Build history of the part. All positions in model axes, mm. Give positions to 0.01 mm unless a question says otherwise; leave off trailing zeros. Loops run counter-clockwise (first coordinate to the right, second up) from the corner with the lowest first, then second, coordinate; pieces in that order, holes last.
1) Wall check: line 1 (Z direction, x = 1.25, y = -9); line 2 (Y direction, x = 0.9, z = 7.75). Give the ranges that are in metal, low to high.
2) Flat gauge pins, fed straight in: P1, Ø3.5, axis at y = -9, z = -9, coming from the -X side; P2, Ø1.8, axis at y = 9, z = 9, coming from the +X side (3 decimals). Where does each tip first touch, or does it go through?
3) Band-saw the part on A-A on y = 9. List the corners of the cut face in (x, z).
4) Band-saw the part on C-C on x = 0.35. List the corners of the cut face in (y, z).
5) Two-plate mould, pull along Z, no slides. Class faces 1 (the flat face through (1.7, 0, 0)), 2 (the cylindrical face through (0.8, 7.8, 9.9)), 3 (the flat face through (1, 0, -11.5)): +Z half, -Z half, draft (parallel to the pull), parting line (faces both ways), or undercut.
Autodesk Inventor part; units mm, degrees
ref_plane "YZ Plane" through (0, 0, 0) normal (1, 0, 0) x (0, 1, 0)
ref_plane "XZ Plane" through (0, 0, 0) normal (0, 1, 0) x (-1, 0, 0)
ref_plane "XY Plane" through (0, 0, 0) normal (0, 0, 1) x (1, 0, 0)
sketch "Sketch1" plane through (0, 0, 0) normal (1, 0, 0) x (0, 1, 0)
  line L0 (11.5, 11.5) -> (-11.5, 11.5)
  line L1 (-11.5, 11.5) -> (-11.5, -11.5)
  line L2 (-11.5, -11.5) -> (11.5, -11.5)
  line L3 (11.5, -11.5) -> (11.5, 11.5)
  line L4 (11.5, 11.5) -> (-11.5, -11.5) construction
  line L5 (-11.5, 11.5) -> (11.5, -11.5) construction
  line L6 (11.5, 11.5) -> (11.5, 9)
  line L7 (11.5, 9) -> (9, 9)
  circle A0 centre (9, 9) radius 1.5
  line L8 (11.5, 0) -> (-11.5, 0)
  line L9 (0, 11.5) -> (0, -11.5)
  line L10 (11.5, -11.5) -> (-11.5, 11.5) construction
  line L11 (11.5, -9) -> (9, -9)
  circle A1 centre (9, -9) radius 1.5
  circle A2 centre (-9, 9) radius 1.5
  circle A3 centre (-9, -9) radius 1.5
  point P0 (0, 0)
  dimension "d0" = 23
  dimension "d1" = 23
  dimension "d2" = 2.5
  dimension "d3" = 2.5
  dimension "d4" = 3
extrude "Extrusion1" add sketch "Sketch1" along normal blind 1.7
ref_plane "Work Plane1" through (0, 0, 11.5) normal (0, 1, 0) x (1, 0, 0)
ref_plane "Work Plane2" through (0, -11.5, 0) normal (0, 0, -1) x (-1, 0, 0)
properties part number "magentic_encoder_modell"
Findings below:
1. line 1: z = -11.5 to -10.5, -7.5 to 7.5, 10.5 to 11.5
1. line 2: y = -11.5 to -9.83, -8.17 to 8.17, 9.83 to 11.5
2. P1: stops at x = 0
2. P2: passes through
3. outline: (0, -11.5) - (1.7, -11.5) - (1.7, -10.5) - (0, -10.5) - close; (0, -7.5) - (1.7, -7.5) - (1.7, 7.5) - (0, 7.5) - close; (0, 10.5) - (1.7, 10.5) - (1.7, 11.5) - (0, 11.5) - close
4. outline: (-11.5, -11.5) - (11.5, -11.5) - (11.5, 11.5) - (-11.5, 11.5) - close; hole circle Ø3 at (-9, -9); hole circle Ø3 at (-9, 9); hole circle Ø3 at (9, -9); hole circle Ø3 at (9, 9)
5. face 1: draft
5. face 2: undercut
5. face 3: -Z half
